```python
from build123d import *

# Parameters (mm, degrees)
SKETCH1_R           = 8
SKETCH1_R_2         = 6
BOSS_EXTRUDE2_DEPTH = 5
BOSS_EXTRUDE3_START = 4
SKETCH1_4_R         = 8
SKETCH1_4_R_2       = 6
BOSS_EXTRUDE3_DEPTH = 4
SKETCH1_8_R         = 8
SKETCH1_8_R_2       = 6
BOSS_EXTRUDE4_DEPTH = 4
SKETCH1_9_R         = 8
SKETCH1_9_R_2       = 6
BOSS_EXTRUDE5_DEPTH = 5
SKETCH1_10_R        = 8
BOSS_EXTRUDE6_DEPTH = 4
BOSS_EXTRUDE7_DEPTH = 2
SKETCH2_R           = 1.5
CUT_EXTRUDE1_DEPTH  = 74
FILLET2_R           = 1


with BuildPart() as part:
    # Sketch1 → Boss-Extrude2 (new body)
    with BuildSketch(Plane.XY):
        with Locations((0, 18)):
            Circle(SKETCH1_R)
        with Locations((0, 18)):
            Circle(SKETCH1_R_2, mode=Mode.SUBTRACT)
    extrude(amount=-BOSS_EXTRUDE2_DEPTH)

    # Sketch1<4> → Boss-Extrude3 (add)
    with BuildSketch(Plane.XY.offset(BOSS_EXTRUDE3_START)):
        with Locations((0, 18)):
            Circle(SKETCH1_4_R)
        with Locations((0, 18)):
            Circle(SKETCH1_4_R_2, mode=Mode.SUBTRACT)
    extrude(amount=-BOSS_EXTRUDE3_DEPTH)



with BuildPart() as body_2:
    # Sketch1<8> → Boss-Extrude4 (new body)
    with BuildSketch(Plane.XY):
        Circle(SKETCH1_8_R)
        Circle(SKETCH1_8_R_2, mode=Mode.SUBTRACT)
    extrude(amount=-BOSS_EXTRUDE4_DEPTH)

    # Sketch1<9> → Boss-Extrude5 (add)
    with BuildSketch(Plane.XY):
        Circle(SKETCH1_9_R)
        Circle(SKETCH1_9_R_2, mode=Mode.SUBTRACT)
    extrude(amount=BOSS_EXTRUDE5_DEPTH)


with BuildPart() as part_1:
    add(part.part)

    add(body_2.part)  # Boss-Extrude6 merges body 2
    # Sketch1<10> → Boss-Extrude6 (add, symmetric)
    with BuildSketch(Plane.XY):
        with BuildLine():
            ThreePointArc((-8, 27.856406461), (0, 30), (8, 27.856406461))
            ThreePointArc((8, 27.856406461), (9.464101615, 26.392304845), (10, 24.392304845))
            Line((10, 24.392304845), (10, 0))
            ThreePointArc((10, 0), (10.826586639, -2.435045716), (12.96472382, -3.863703305))
            Line((12.96472382, -3.863703305), (30.521723645, -8.56808723))
            ThreePointArc((30.521723645, -8.56808723), (33.079490803, -10.673939697), (33.172253398, -13.985764352))
            ThreePointArc((33.172253398, -13.985764352), (0, -36), (-33.172253398, -13.985764352))
            ThreePointArc((-33.172253398, -13.985764352), (-33.079490803, -10.673939697), (-30.521723645, -8.56808723))
            Line((-30.521723645, -8.56808723), (-12.96472382, -3.863703305))
            ThreePointArc((-12.96472382, -3.863703305), (-10.826586639, -2.435045716), (-10, 0))
            Line((-10, 0), (-10, 24.392304845))
            ThreePointArc((-10, 24.392304845), (-9.464101615, 26.392304845), (-8, 27.856406461))
        make_face()
        with Locations((0, 18)):
            Circle(SKETCH1_10_R, mode=Mode.SUBTRACT)
        Circle(SKETCH1_10_R, mode=Mode.SUBTRACT)
        with BuildLine():
            ThreePointArc((12.188266684, -6.761480784), (9.876608994, -6.714952527), (7.808142843, -7.748090432))
            ThreePointArc((7.808142843, -7.748090432), (0, -11), (-7.808142843, -7.748090432))
            ThreePointArc((-7.808142843, -7.748090432), (-9.876608994, -6.714952527), (-12.188266684, -6.761480784))
            Line((-12.188266684, -6.761480784), (-29.74526651, -11.465864709))
            ThreePointArc((-29.74526651, -11.465864709), (-30.384708299, -11.992327826), (-30.407898948, -12.820283989))
            ThreePointArc((-30.407898948, -12.820283989), (0, -33), (30.407898948, -12.820283989))
            ThreePointArc((30.407898948, -12.820283989), (30.384708299, -11.992327826), (29.74526651, -11.465864709))
            Line((29.74526651, -11.465864709), (12.188266684, -6.761480784))
        make_face(mode=Mode.SUBTRACT)
    extrude(amount=BOSS_EXTRUDE6_DEPTH, both=True)

    # Sketch1<11> → Boss-Extrude7 (add, symmetric)
    with BuildSketch(Plane.XY):
        with BuildLine():
            Line((12.188266684, -6.761480784), (29.74526651, -11.465864709))
            ThreePointArc((29.74526651, -11.465864709), (30.384708299, -11.992327826), (30.407898948, -12.820283989))
            ThreePointArc((30.407898948, -12.820283989), (0, -33), (-30.407898948, -12.820283989))
            ThreePointArc((-30.407898948, -12.820283989), (-30.384708299, -11.992327826), (-29.74526651, -11.465864709))
            Line((-29.74526651, -11.465864709), (-12.188266684, -6.761480784))
            ThreePointArc((-12.188266684, -6.761480784), (-9.876608994, -6.714952527), (-7.808142843, -7.748090432))
            ThreePointArc((-7.808142843, -7.748090432), (0, -11), (7.808142843, -7.748090432))
            ThreePointArc((7.808142843, -7.748090432), (9.876608994, -6.714952527), (12.188266684, -6.761480784))
        make_face()
    extrude(amount=BOSS_EXTRUDE7_DEPTH, both=True)

    # Sketch2 → Cut-Extrude1 (cut, symmetric)
    with BuildSketch(Plane(origin=(0, 0, 0), x_dir=(0, 0, -1), z_dir=(1, 0, 0))):
        with Locations((-0.5, 18)):
            Circle(SKETCH2_R)
        with Locations((-0.5, 0)):
            Circle(SKETCH2_R)
    extrude(amount=CUT_EXTRUDE1_DEPTH, both=True, mode=Mode.SUBTRACT)

    # Fillet2
    fillet2_edges = [part_1.edges().sort_by_distance(p)[0] for p in [
        (20.966766597, -9.113672746, 2),
        (0, -11, 2),
        (-9.876608994, -6.714952527, 2),
        (0, -33, 2),
        (30.384708299, -11.992327826, 2),
        (9.876608994, -6.714952527, 2),
        (-20.966766597, -9.113672746, 2),
        (-30.384708299, -11.992327826, 2),
    ]]
    fillet(fillet2_edges, radius=FILLET2_R)


solid = part_1.part
```
Verification items for the finished model (mm, model axes). A direction names the side the tool comes from. Round coordinates to 2 decimals unless told otherwise and drop trailing zeros. Order: outer loops, then holes, each group sorted by start corner. A loop starts at its lowest first (then second) coordinate and runs counter-clockwise, first axis right, second up.
1) Depth check by flat-ended pin: pin 1 (21 mm diameter, centred on x = -1.5, y = -15.5, fed in from -Z); pin 2 (2.5 mm diameter, centred on y = 18, z = 0.5, fed in from +X); pin 3 (3.5 mm diameter, centred on y = 18, z = 0.5, fed in from +X); pin 4 (5 mm diameter, centred on y = 0, z = 0.5, fed in from +X). Enter the tip coordinate at first touch or a pass-through.
Geometry says:
pin 1: stops at z = -4
pin 2: passes through
pin 3: stops at x = 10
pin 4: stops at x = 10.88
2) Cross-section at A-A, the plane x = 0. Give the number of separate pieces and of enclosed holes in the cut face, plus the area to 3 significant figures.
Geometry says:
separate pieces: 3
enclosed holes: 0
area: 256 mm2
3) Material ranges on line 1 (Y direction, x = -7.5, z = 1.25); line 2 (Y direction, x = -9.15, z = 0.5); line 3 (Y direction, x = 3.5, z = 2.5), recorded low to high.
Geometry says:
line 1: y = -35.21 to -1.3, 1.3 to 16.7, 19.3 to 28.13
line 2: y = -34.82 to -1.5, 1.5 to 16.5, 19.5 to 26.86
line 3: y = -35.83 to -32.68, -10.57 to -4.87, 4.87 to 13.13, 22.87 to 29.61
4) Tool access check on faces 1 (the cylindrical face through (0.1, -11, 3.5)), 2 (the flat face through (21.62, -6.183, 0.056)), 3 (the flat face through (0, -20, -2)). Record the directions out of +Z, -Z, +X, -X, +Y, -Y that give a thin tool (end or side, any length) a straight path to the whole face; none if there is none.
Geometry says:
face 1: +Z
face 2: +Z, -Z, +X, +Y
face 3: -Z
5) Draft check along X on faces 4 (the cylindrical face through (-9.845, -6.722, -2.986)), 5 (the cylindrical face through (-9.479, 26.367, 0.056)), 6 (the cylindrical face through (-8.02, -1.33, -0.19)), 7 (the cylindrical face through (33.058, -10.631, 0.056)). Enter one of: +X half, -X half, draft (parallel to the pull), parting line (faces both ways), or undercut.
Geometry says:
face 4: undercut
face 5: -X half
face 6: draft
face 7: +X half
6) Cross-section at B-B, the plane y = 18. Record the cut outline in (x, z).
Geometry says:
outline: (-10, -4) - (-8, -4) - (-8, -5) - (-6, -5) - (-6, -1) - (-10, -1) - close; (-10, 2) - (-6, 2) - (-6, 4) - (-10, 4) - close; (6, -5) - (8, -5) - (8, -4) - (10, -4) - (10, -1) - (6, -1) - close; (6, 2) - (10, 2) - (10, 4) - (6, 4) - close
